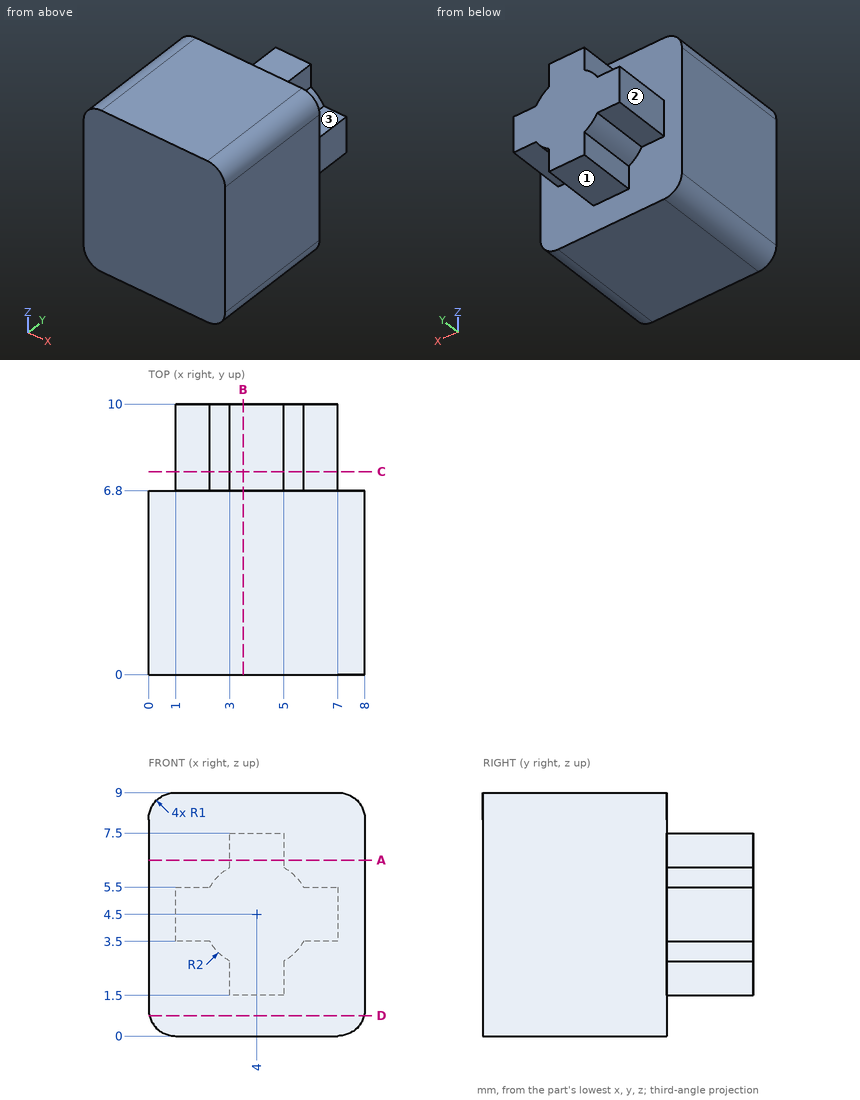
Answer from the drawing. Dimensions are ordinates in mm from the lowest x, y and z of the part. A direction names the side the tool comes from. Coordinates: 2 decimals unless noted, no trailing zeros. Order: outer loops, then holes, each group sorted by start corner. A loop starts at its lowest first (then second) coordinate and runs counter-clockwise, first axis right, second up. Notation, with made-up numbers: M -20.5,54.25 L 12.5,54.25 A27 cw 12.5,72.25 Z; hole C -24,53.25 d11. An arc over 180 degrees is marked long. Put each result on its own line as item: value. Start each with the question number.
Item 1: Section C-C, the plane y = 7.5 is taken. Determine the outline of the cut face in (x, z), plus the area to 3 significant figures.
Item 2: Section D-D, the plane z = 0.75 is taken. Determine the outline of the cut face in (x, y).
Item 3: Section A-A, the plane z = 6.5 is taken. Determine the outline of the cut face in (x, y).
Item 4: Section B-B, the plane x = 3.5 is taken. Determine the outline of the cut face in (y, z), plus the area to 3 significant figures.
Item 5: For the marked faces 1, 2 and 3, determine the directions among +Z, -Z, +X, -X, +Y, -Y from which every point of the face is accessible in a straight line to the end or side of a thin tool.
Item 6: Given pin 1 Ø0.6 at (x, y) = (6, 9) entering from -Z; pin 2 Ø2 at (y, z) = (8, 4) entering from +X; pin 3 Ø1.4 at (x, y) = (2, 8) entering from -Z, each flat-ended and moving along its own axis, determine where each tip first touches the part or whether it passes through.
Item 7: Consider probe 1 along Y at (x, z) = (6.75, 2.5); probe 2 along X at (y, z) = (9, 3.75); probe 3 along Z at (x, y) = (4.5, 9.25). Determine where each line is inside the solid, lowest interval first. Write a range as [from, to].
Computed:
1. outline: M 1,3.5 L 2.27,3.5 A2 ccw 3,2.77 L 3,1.5 L 5,1.5 L 5,2.77 A2 ccw 5.73,3.5 L 7,3.5 L 7,5.5 L 5.73,5.5 A2 ccw 5,6.23 L 5,7.5 L 3,7.5 L 3,6.23 A2 ccw 2.27,5.5 L 1,5.5 Z
1. area: 21.3 mm2
2. outline: M 0.03,0 L 7.97,0 L 7.97,6.8 L 0.03,6.8 Z
3. outline: M 0,0 L 8,0 L 8,6.8 L 5,6.8 L 5,10 L 3,10 L 3,6.8 L 0,6.8 Z
4. outline: M 0,0 L 6.8,0 L 6.8,1.5 L 10,1.5 L 10,7.5 L 6.8,7.5 L 6.8,9 L 0,9 Z
4. area: 80.4 mm2
5. face 1: -Z, +X, -X, +Y
5. face 2: +Z, -Z, -X, +Y
5. face 3: +Z, +X, +Y
6. pin 1: stops at z = 3.45
6. pin 2: stops at x = 7
6. pin 3: stops at z = 2.98
7. probe 1: y = [0, 6.8]
7. probe 2: x = [1, 7]
7. probe 3: z = [1.5, 7.5]
